Verification items for the finished model (mm, model axes). Face numbers are marked on the shaded views. A direction names the side the tool comes from. Round coordinates to 2 decimals unless told otherwise and drop trailing zeros. One line per item, written item: value. Start each with the question number.
Item 1: Tool access check on the marked faces 4 and 5. Record the directions out of +Z, -Z, +X, -X, +Y, -Y that give a thin tool (end or side, any length) a straight path to the whole face; none if there is none.
Item 2: Gauge pin test, flat ends, axial feed: pin 1 (6 mm diameter, centred on x = 31, y = -24.5, fed in from +Z); pin 2 (3 mm diameter, centred on x = -5, z = 3.5, fed in from +Y); pin 3 (12 mm diameter, centred on y = 10.5, z = 14, fed in from -X). Record the tip position at first contact, or that the pin passes through.
Item 3: Draft check along Y on the marked faces 1, 2 and 3. Enter one of: +Y half, -Y half, draft (parallel to the pull), parting line (faces both ways), or undercut.
Item 4: Thickness scan on probe 1 along X at (y, z) = (4.5, 3.5); probe 2 along Z at (x, y) = (38.5, 3.5); probe 3 along Z at (x, y) = (-22.5, -2.5). Record the ranges inside material, lowest first. Write a range as from..to.
from build123d import *

# Parameters (mm, degrees)
FILLET2_R           = 5.08
SKETCH3_R           = 4.826
BOSS_EXTRUDE1_DEPTH = 12.7
SKETCH5_R           = 4.826
BOSS_EXTRUDE2_DEPTH = 12.7


with BuildPart() as part:
    # Sketch1 → Revolve2 (revolve)
    with BuildSketch(Plane.XY):
        with BuildLine():
            Line((45.524615385, -0.976923077), (45.524615385, 24.423076923))
            Line((45.524615385, 24.423076923), (20.124615385, 24.423076923))
            ThreePointArc((20.124615385, 24.423076923), (-14.744833443, 27.875832785), (-48.26, 38.1))
            Line((-48.26, 38.1), (-50.8, 38.1))
            Line((-50.8, 38.1), (-76.2, 38.1))
            Line((-76.2, 38.1), (-76.2, 0))
            Line((-76.2, 0), (45.524615385, -0.976923077))
        make_face()
    revolve(axis=Axis((45.524615385, -0.976923077, 0), (-0.9999677957684845, 0.008025423722058495, 0)))

    # Fillet2
    fillet2_edges = [part.edges().sort_by_distance(p)[0] for p in [
        (45.116936989, -26.37365118, 0),
    ]]
    fillet(fillet2_edges, radius=FILLET2_R)

    # Chamfer1: read off the stored shape, not the designer's step
    # Chamfer1 outline → Chamfer1 (revolve, cut)
    with BuildSketch(Plane(origin=(-0.004907846, -0.611517594, 0), x_dir=(0.008025423722058226, 0.9999677957684845, 0), z_dir=(0, 0, -1))):
        Polygon((30.479018415, -76.442160953), (30.479018415, -76.503314681), (38.098773019, -76.503314681), (38.323003358, -48.564214468), (38.323003358, -48.368371001), (38.243376135, -48.368371001), align=None)
    revolve(axis=Axis((-0.004907846, -0.611517594, 0), (0.9999677957684845, -0.008025423722058226, 0)), mode=Mode.SUBTRACT)

    # Sketch3 → Boss-Extrude1 (add, symmetric)
    with BuildSketch(Plane(origin=(-76.2, 0, 0), x_dir=(0, 0, -1), z_dir=(1, 0, 0))):
        with Locations(Location((0, 0, 0), (0, 0, 305.528030249))):
            Circle(SKETCH3_R)
    extrude(amount=BOSS_EXTRUDE1_DEPTH, both=True)

    # Sketch5 → Boss-Extrude2 (add, symmetric)
    with BuildSketch(Plane(origin=(0, -39.37, 0), x_dir=(1, 0, 0), z_dir=(0, 1, 0))):
        with Locations(Location((-36.216917905, 0, 0), (0, 0, 141.940248705))):
            Circle(SKETCH5_R)
    extrude(amount=BOSS_EXTRUDE2_DEPTH, both=True)


solid = part.part
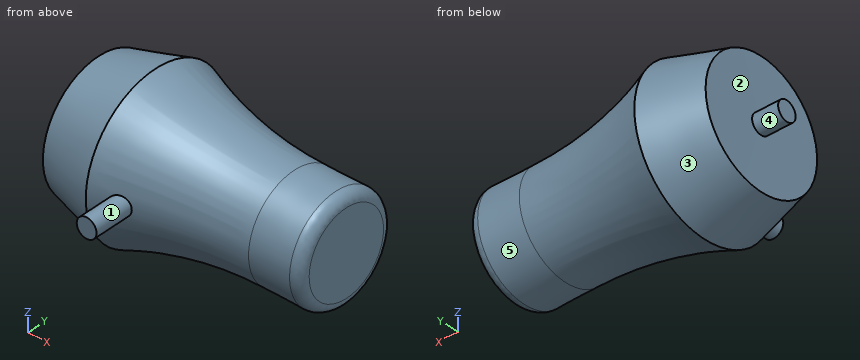
Response values:
1. face 4: -X
1. face 5: none
2. pin 1: stops at z = 14.61
2. pin 2: stops at y = 26.26
2. pin 3: stops at x = -76.31
3. face 1: draft
3. face 2: undercut
3. face 3: parting line
4. probe 1: x = -76.21..45.52
4. probe 2: z = -24.96..24.96
4. probe 3: z = -29.91..29.91
